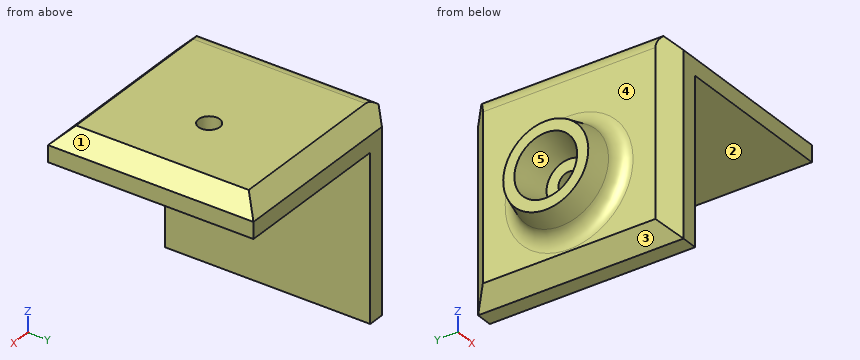
```python
from build123d import *

# Parameters (mm, degrees)
BOSS_EXTRUDE1_DEPTH = 50
SKETCH2_R           = 2.6
CUT_EXTRUDE1_DEPTH  = 81.024996095
SKETCH3_R           = 2.6
CUT_EXTRUDE2_DEPTH  = 81.024996095
SKETCH4_R           = 12.5
SKETCH4_R_2         = 5.5
BOSS_EXTRUDE2_DEPTH = 8
BOSS_EXTRUDE2_DRAFT = 15
FILLET1_R           = 4
CHAMFER1_SIZE       = 4
FILLET2_R           = 4


with BuildPart() as part:
    # Sketch1 → Boss-Extrude1 (new body)
    with BuildSketch(Plane(origin=(0, 0, 0), x_dir=(1, 0, 0), z_dir=(0, 1, 0))):
        Polygon((-8, 40), (0, 40), (0, 0), (40, 0), (40, -8), (-8, -8), align=None)
    extrude(amount=BOSS_EXTRUDE1_DEPTH)

    # Sketch2 → Cut-Extrude1 (cut, through all)
    with BuildSketch(Plane.ZY.offset(8)):
        with Locations((-20, 25)):
            Circle(SKETCH2_R)
    extrude(amount=-CUT_EXTRUDE1_DEPTH, mode=Mode.SUBTRACT)

    # Sketch3 → Cut-Extrude2 (cut, through all)
    with BuildSketch(Plane.XY.offset(8)):
        with Locations((20, 25)):
            Circle(SKETCH3_R)
    extrude(amount=-CUT_EXTRUDE2_DEPTH, mode=Mode.SUBTRACT)


with BuildPart() as boss_extrude2_tool:
    # Sketch4 → Boss-Extrude2 (with draft: the straight prism first)
    with BuildSketch(Plane.ZY.offset(8)):
        with Locations((-20, 25)):
            Circle(SKETCH4_R)
        with Locations((-20, 25)):
            Circle(SKETCH4_R_2, mode=Mode.SUBTRACT)
    extrude(amount=BOSS_EXTRUDE2_DEPTH)
    # Boss-Extrude2: the draft: its side faces are tilted about the plane it starts from
    boss_extrude2_sides = [boss_extrude2_tool.faces().sort_by_distance(p)[0] for p in [
        (-12, 25, -32.5),
        (-12, 25, -25.5),
    ]]
    draft(boss_extrude2_sides, Plane.ZY.offset(8), BOSS_EXTRUDE2_DRAFT)


with BuildPart() as part_1:
    add(part.part)

    # Boss-Extrude2: add boss_extrude2_tool
    add(boss_extrude2_tool.part)

    # Fillet1
    fillet1_edges = [part_1.edges().sort_by_distance(p)[0] for p in [
        (-8, 25, -32.5),
    ]]
    fillet(fillet1_edges, radius=FILLET1_R)

    # Chamfer1
    chamfer1_edges = [part_1.edges().sort_by_distance(p)[0] for p in [
        (-8, 25, -40),
        (40, 25, 8),
        (-8, 50, -16),
        (16, 0, 8),
        (-8, 0, -16),
        (16, 50, 8),
    ]]
    chamfer(chamfer1_edges, length=CHAMFER1_SIZE)

    # Fillet2
    fillet2_edges = [part_1.edges().sort_by_distance(p)[0] for p in [
        (-8, 25, 8),
    ]]
    fillet(fillet2_edges, radius=FILLET2_R)


solid = part_1.part
```
Here's how the part is built. I have some questions about the finished solid (model axes, mm). Face numbers are marked on the shaded views. A direction names the side the tool comes from. Coordinates: 2 decimals unless noted, no trailing zeros. Order: outer loops, then holes, each group sorted by start corner. A loop starts at its lowest first (then second) coordinate and runs counter-clockwise, first axis right, second up. Notation, with made-up numbers: (-7.5, 3) -> (50.5, 3) arc R8 cw to (50.5, 17) -> close; hole circle Ø7 at (59.25, -11.5). An arc over 180 degrees is marked (long way). Return JSON: item names as keys, results as strings.
1) Thinking about a two-plate mould opening in Z: for the marked faces 3, 4 and 5, which applies, +Z half, -Z half, draft (parallel to the pull), parting line (faces both ways), or undercut?
Conclusion:
{"face 3": "-Z half", "face 4": "draft", "face 5": "undercut"}
2) On a 3-axis mill with a long thin cutter (end or side, diameter ignored), from which of +Z, -Z, +X, -X, +Y, -Y can I reach the whole of each face in a straight line? I mean the marked faces 1 and 2. Say none if no direction works.
Conclusion:
{"face 1": "+Z, +X, +Y, -Y", "face 2": "-Z, +X, +Y, -Y"}
3) I'm going to push flat-ended pins straight in: P1, Ø3, axis at x = 24.5, y = 20.5, coming from the -Z side; P2, Ø6, axis at y = 42, z = -7, coming from the +X side. Where does each tip first touch, or does it pass through?
Conclusion:
{"P1": "stops at z = 0", "P2": "stops at x = 0"}
4) If we section it at D-D on y = 43: List the corners of the cut face in (x, z) for me, plus the area to 3 significant figures.
Conclusion:
{"outline": "(-8, -36) -> (-4, -40) -> (0, -40) -> (0, 0) -> (40, 0) -> (40, 4) -> (36, 8) -> (-4, 8) arc R4 ccw to (-8, 4) -> close", "area": "685 mm²"}
5) If we section it at C-C on y = 25: List the corners of the cut face in (x, z) for me, plus the area to 3 significant figures.
Conclusion:
{"outline": "(-16, -30.36) -> (-10.96, -31.71) arc R4 cw to (-8, -35.57) -> (-8, -36) -> (-4, -40) -> (0, -40) -> (0, -22.6) -> (-8, -22.6) -> (-8, -25.5) -> (-16, -27.64) -> close; (-16, -12.36) -> (-8, -14.5) -> (-8, -17.4) -> (0, -17.4) -> (0, 0) -> (17.4, 0) -> (17.4, 8) -> (-4, 8) arc R4 ccw to (-8, 4) -> (-8, -4.43) arc R4 cw to (-10.96, -8.29) -> (-16, -9.64) -> close; (22.6, 0) -> (40, 0) -> (40, 4) -> (36, 8) -> (22.6, 8) -> close", "area": "683 mm²"}
6) If we section it at A-A on z = -20: List the corners of the cut face in (x, y) for me, plus the area to 3 significant figures.
Conclusion:
{"outline": "(-16, 14.64) -> (-10.96, 13.29) arc R4 cw to (-8, 9.43) -> (-8, 4) -> (-4, 0) -> (0, 0) -> (0, 22.4) -> (-8, 22.4) -> (-8, 19.5) -> (-16, 17.36) -> close; (-16, 32.64) -> (-8, 30.5) -> (-8, 27.6) -> (0, 27.6) -> (0, 50) -> (-4, 50) -> (-8, 46) -> (-8, 40.57) arc R4 cw to (-10.96, 36.71) -> (-16, 35.36) -> close", "area": "424 mm²"}
7) If I drill on probe 1 along Y at (x, z) = (-2.75, -20); probe 2 along Z at (x, y) = (8, 17.5); probe 3 along X at (y, z) = (29, -28), over which ranges is the centre line in solid material (lowest first)?
Conclusion:
{"probe 1": "y = 0 to 22.4, 27.6 to 50", "probe 2": "z = 0 to 8", "probe 3": "x = -16 to 0"}
8) If we section it at B-B on x = 20: List the corners of the cut face in (y, z) for me, plus the area to 3 significant figures.
Conclusion:
{"outline": "(0, 0) -> (22.4, 0) -> (22.4, 8) -> (4, 8) -> (0, 4) -> close; (27.6, 0) -> (50, 0) -> (50, 4) -> (46, 8) -> (27.6, 8) -> close", "area": "342 mm²"}
